```python
from build123d import *

# Parameters (mm, degrees)
SKIZZE1_W                       = 25
SKIZZE1_H                       = 15
SKIZZE1_R                       = 4
AUFSATZ_LINEAR_AUSTRAGEN1_DEPTH = 40
SCHNITT_LINEAR_START            = -15
SCHNITT_LINEAR_AUSTRAGEN1_DEPTH = 71
M3_GEWINDEBOHRUNG1_D            = 2.5
VERRUNDUNG2_R                   = 2
SKIZZE5_W                       = 17.099513742
SKIZZE5_H                       = 10
SCHNITT_LINEAR_AUSTRAGEN2_DEPTH = 13
AUFSATZ_LINEAR_START            = -15
SKIZZE6_R                       = 4
SKIZZE6_R_2                     = 2.5
AUFSATZ_LINEAR_AUSTRAGEN2_DEPTH = 15
VERRUNDUNG5_R                   = 5
VERRUNDUNG6_R                   = 2
VERRUNDUNG7_R                   = 1.5


# Some blends are built 0.0001 mm under size
with BuildPart() as part:
    # Skizze1 → Aufsatz-Linear austragen1 (new body)
    with BuildSketch(Plane(origin=(0, 0, 0), x_dir=(1, 0, 0), z_dir=(0, 1, 0))):
        with Locations((4.5, 0)):
            Rectangle(SKIZZE1_W, SKIZZE1_H)
        with Locations(Location((0, 0, 0), (0, 0, 270))):
            Circle(SKIZZE1_R, mode=Mode.SUBTRACT)
    extrude(amount=AUFSATZ_LINEAR_AUSTRAGEN1_DEPTH)

    # Skizze2 → Schnitt-Linear austragen1 (cut)
    with BuildSketch(Plane(origin=(0, 40, 0), x_dir=(1, 0, 0), z_dir=(0, 1, 0)).offset(SCHNITT_LINEAR_START)):
        with BuildLine():
            Line((0, 1.5), (23.752899364, 1.5))
            ThreePointArc((23.752899364, 1.5), (25.252899364, 0), (23.752899364, -1.5))
            Line((23.752899364, -1.5), (0, -1.5))
            ThreePointArc((0, -1.5), (-1.5, 0), (0, 1.5))
        make_face()
    extrude(amount=-SCHNITT_LINEAR_AUSTRAGEN1_DEPTH, mode=Mode.SUBTRACT)

    # M3 Gewindebohrung1 (through all)
    with Locations(Plane.XY.offset(7.5)):
        with Locations((12, 5)):
            Hole(M3_GEWINDEBOHRUNG1_D / 2)

    # Verrundung2
    verrundung2_edges = [part.edges().sort_by_distance(p)[0] for p in [
        (3.708099244, 12.5, 1.5),
        (3.708099244, 12.5, -1.5),
    ]]
    fillet(verrundung2_edges, radius=VERRUNDUNG2_R)

    # Skizze5 → Schnitt-Linear austragen2 (cut, symmetric)
    with BuildSketch(Plane.XY):
        with Locations((-3.960992506, 20)):
            Rectangle(SKIZZE5_W, SKIZZE5_H)
    extrude(amount=SCHNITT_LINEAR_AUSTRAGEN2_DEPTH, both=True, mode=Mode.SUBTRACT)

    # Skizze6 → Aufsatz-Linear austragen2 (add)
    with BuildSketch(Plane(origin=(0, 40, 0), x_dir=(1, 0, 0), z_dir=(0, 1, 0)).offset(AUFSATZ_LINEAR_START)):
        Circle(SKIZZE6_R)
        with Locations(Location((0, 0, 0), (0, 0, 270))):
            Circle(SKIZZE6_R_2, mode=Mode.SUBTRACT)
    extrude(amount=AUFSATZ_LINEAR_AUSTRAGEN2_DEPTH)

    # Verrundung5
    # the kernel refuses this fillet: 5 mm, written as the material it takes off along each edge
    with BuildSketch(Plane(origin=(17, 40, -20), x_dir=(0, -1, 0), z_dir=(0, 0, 1)), Plane(origin=(-8, 0, 20), x_dir=(1, 0, 0), z_dir=(0, 0, -1)), Plane(origin=(-8, 15, 20), x_dir=(0, -1, 0), z_dir=(0, 0, -1))) as verrundung5_piece_1:
        with BuildLine():
            CenterArc((VERRUNDUNG5_R, -VERRUNDUNG5_R), VERRUNDUNG5_R, 90, 90)
            Line((0, -VERRUNDUNG5_R), (0, 0))
            Line((0, 0), (VERRUNDUNG5_R, 0))
        make_face()
    extrude(amount=40, mode=Mode.SUBTRACT)
    with BuildSketch(Plane(origin=(17, 0, -20), x_dir=(-1, 0, 0), z_dir=(0, 0, 1)), Plane(origin=(17, 0, -11), x_dir=(-1, 0, 0), z_dir=(0, 0, 1))) as verrundung5_piece_2:
        with BuildLine():
            CenterArc((VERRUNDUNG5_R, -VERRUNDUNG5_R), VERRUNDUNG5_R, 90, 90)
            Line((0, -VERRUNDUNG5_R), (0, 0))
            Line((0, 0), (VERRUNDUNG5_R, 0))
        make_face()
    extrude(amount=31, mode=Mode.SUBTRACT)
    with BuildSketch(Plane(origin=(-8, 40, 20), x_dir=(1, 0, 0), z_dir=(0, 0, -1)), Plane(origin=(-8, 25, -20), x_dir=(1, 0, 0), z_dir=(0, 0, 1))) as verrundung5_piece_3:
        with BuildLine():
            CenterArc((VERRUNDUNG5_R, VERRUNDUNG5_R), VERRUNDUNG5_R, 180, 90)
            Line((0, VERRUNDUNG5_R), (0, 0))
            Line((0, 0), (VERRUNDUNG5_R, 0))
        make_face()
    extrude(amount=40, mode=Mode.SUBTRACT)

    # Verrundung6
    verrundung6_edges = [part.edges().sort_by_distance(p)[0] for p in [
        (-8, 7.5, 7.5),
        (-8, 7.5, -7.5),
        (-8, 32.5, 7.5),
        (0.794382183, 25, 7.5),
        (4.5, 0, 7.5),
        (17, 20, 7.5),
        (4.5, 40, 7.5),
        (15.535533906, 1.464466094, 7.5),
        (15.535533906, 38.535533906, 7.5),
        (-6.535533906, 38.535533906, 7.5),
        (-6.535533906, 26.464466094, 7.5),
        (-6.535533906, 13.535533906, 7.5),
        (-6.535533906, 1.464466094, 7.5),
        (4.5, 0, -7.5),
        (-8, 32.5, -7.5),
        (4.5, 40, -7.5),
        (17, 20, -7.5),
        (0.794382183, 15, -7.5),
        (15.535533906, 1.464466094, -7.5),
        (15.535533906, 38.535533906, -7.5),
        (-6.535533906, 38.535533906, -7.5),
        (-6.535533906, 26.464466094, -7.5),
        (-6.535533906, 13.535533906, -7.5),
        (-6.535533906, 1.464466094, -7.5),
        (0.794382183, 25, -7.5),
        (4.588764365, 20, 7.5),
        (4.588764365, 20, -7.5),
        (0.794382183, 15, 7.5),
    ]]
    fillet(verrundung6_edges, radius=VERRUNDUNG6_R)

    # Verrundung7
    verrundung7_edges = [part.edges().sort_by_distance(p)[0] for p in [
        (4.730717229, 25, 1.505095884),
        (4.730717229, 25, -1.505095884),
        (10.936698586, 25, 1.5),
        (10.936698586, 25, -1.5),
    ]]
    fillet(verrundung7_edges, radius=VERRUNDUNG7_R - 0.0001)  # a hair under: the kernel refuses the full size


solid = part.part
```
Could you check a few things on this model? Use its own coordinates, in mm. A direction names the side the tool comes from. Coordinates: 2 decimals unless noted, no trailing zeros. Loops run counter-clockwise (first coordinate to the right, second up) from the corner with the lowest first, then second, coordinate; pieces in that order, holes last. Notation, with made-up numbers: M 0.5,-9 L 43.5,-9 A9 ccw 43.5,4 Z; hole C -5.75,18.5 d7. An arc over 180 degrees is marked long. Put each result on its own line as item: value. Start each with the question number.
(1) I need wall thicknesses on line 1 (Y direction, x = 12, z = 5.35); line 2 (Z direction, x = 11, y = 2); line 3 (Y direction, x = -3, z = -2). Which ranges of each line are inside material? Lowest first, please. Write a range as from..to.
(2) Suppose I cut it at A-A on y = 16. Please give me the cut outline in (x, z).
(3) Suppose I cut it at C-C on x = -0.75. Please give me the cut outline in (y, z).
(4) Will these pins go through, and if not, where does the flat tip stop? P1, Ø6, axis at y = 19, z = 4, coming from the -X side; P2, Ø7, axis at x = 0, z = 0, coming from the -Y side; P3, Ø3, axis at x = 0, z = 0, coming from the +Y side.
(5) Thinking about a two-plate mould opening in Y: for faces 1 (the face through (0.8, 14.4, -6.93)), 2 (the face through (4, 40, 0)), 3 (the face through (16.4, 19.79, 6.93)), 4 (the face through (6, 0, -4)), which applies, pulls with the +Y half, pulls with the -Y half, needs draft (parallel to the pull), parting line crosses it, or undercut?
(6) For faces 5 (the face through (-4, 7, 0)), 6 (the face through (0.8, 14.4, 6.93)), 7 (the face through (-7, 27, 0)), which set-ups out of +Z, -Z, +X, -X, +Y, -Y let a thin tool reach every point of the face, with its end or its side?
(7) Suppose I cut it at D-D on y = 24. Please give me the cut outline in (x, z), then the cut area to 3 significant figures.
Solutions:
1. line 1: y = 0..3.75, 6.25..40
1. line 2: z = -7.5..-1.5, 1.5..7.5
1. line 3: y = 25..40
2. outline: M 4.59,-5.5 A2 ccw 6.59,-7.5 L 15,-7.5 A2 ccw 17,-5.5 L 17,-1.5 L 4.87,-1.5 A2 ccw 4.59,-1.52 Z; M 4.59,1.52 A2 ccw 4.87,1.5 L 17,1.5 L 17,5.5 A2 ccw 15,7.5 L 6.59,7.5 A2 ccw 4.59,5.5 Z
3. outline: M 0,-5.5 A2 ccw 2,-7.5 L 13,-7.5 A2 ccw 15,-5.5 L 15,-3.93 L 0,-3.93 Z; M 0,3.93 L 15,3.93 L 15,5.5 A2 ccw 13,7.5 L 2,7.5 A2 ccw 0,5.5 Z; M 25,-5.5 A2 ccw 27,-7.5 L 38,-7.5 A2 ccw 40,-5.5 L 40,-2.38 L 25,-2.38 Z; M 25,2.38 L 40,2.38 L 40,5.5 A2 ccw 38,7.5 L 27,7.5 A2 ccw 25,5.5 Z
4. P1: stops at x = 4.59
4. P2: stops at y = 25
4. P3: passes through
5. face 1: undercut
5. face 2: pulls with the +Y half
5. face 3: needs draft
5. face 4: pulls with the -Y half
6. face 5: -Y
6. face 6: +Z, -X
6. face 7: +Z, -Z, -X
7. outline: M 4.59,-5.5 A2 ccw 6.59,-7.5 L 15,-7.5 A2 ccw 17,-5.5 L 17,-1.41 L 4.87,-1.41 A2.09 ccw 4.59,-1.43 Z; M 4.59,1.43 A2.09 ccw 4.87,1.41 L 17,1.41 L 17,5.5 A2 ccw 15,7.5 L 6.59,7.5 A2 ccw 4.59,5.5 Z
7. area: 148 mm2
